For this review, take the finished solid that the model builds, in its own axes (mm). Face numbers are marked on the shaded views. A direction names the side the tool comes from. Round coordinates to 2 decimals unless told otherwise and drop trailing zeros. Order: outer loops, then holes, each group sorted by start corner. A loop starts at its lowest first (then second) coordinate and runs counter-clockwise, first axis right, second up. Notation, with made-up numbers: M -5,-23.5 L 28,-23.5 A16 cw 28,-8.5 Z; hole C 68,84.5 d1. An arc over 180 degrees is marked long. Use a Markdown table: item, result.
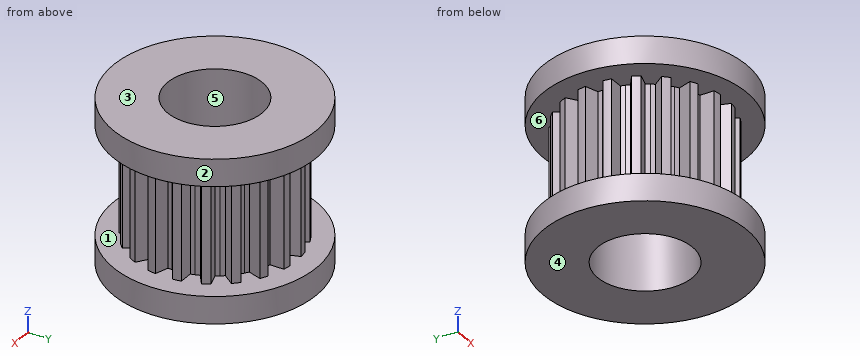
from build123d import *

# Parameters (mm, degrees)
BOSS_EXTRUDE1_DEPTH = 8
SKETCH3_R           = 7.5
BOSS_EXTRUDE2_DEPTH = 2
BOSS_EXTRUDE3_START = 2
SKETCH4_R           = 7.5
BOSS_EXTRUDE3_DEPTH = 2
SKETCH5_R           = 3.5
CUT_EXTRUDE1_DEPTH  = 17.015617378


with BuildPart() as part:
    # Sketch2 → Boss-Extrude1 (new body)
    with BuildSketch(Plane.XY):
        with BuildLine():
            Line((0.323954703, 4.989494298), (0.641126295, 5.965648085))
            ThreePointArc((0.641126295, 5.965648085), (0.93860679, 5.926130044), (1.2337393, 5.871787406))
            Line((1.2337393, 5.871787406), (1.2337393, 4.845398574))
            ThreePointArc((1.2337393, 4.845398574), (1.390142549, 4.802864114), (1.545084972, 4.755282581))
            ThreePointArc((1.545084972, 4.755282581), (1.698403748, 4.702703978), (1.849937763, 4.645183556))
            Line((1.849937763, 4.645183556), (2.453233982, 5.475549564))
            ThreePointArc((2.453233982, 5.475549564), (2.723942998, 5.346039145), (2.987837896, 5.203155264))
            Line((2.987837896, 5.203155264), (2.670666304, 4.227001478))
            ThreePointArc((2.670666304, 4.227001478), (2.806270762, 4.13821754), (2.938926261, 4.045084972))
            ThreePointArc((2.938926261, 4.045084972), (3.068493401, 3.947701641), (3.194836025, 3.846169883))
            Line((3.194836025, 3.846169883), (4.025202033, 4.449466102))
            ThreePointArc((4.025202033, 4.449466102), (4.242640687, 4.242640687), (4.449466102, 4.025202033))
            Line((4.449466102, 4.025202033), (3.846169883, 3.194836025))
            ThreePointArc((3.846169883, 3.194836025), (3.947701641, 3.068493401), (4.045084972, 2.938926261))
            ThreePointArc((4.045084972, 2.938926261), (4.13821754, 2.806270762), (4.227001478, 2.670666304))
            Line((4.227001478, 2.670666304), (5.203155264, 2.987837896))
            ThreePointArc((5.203155264, 2.987837896), (5.346039145, 2.723942998), (5.475549564, 2.453233982))
            Line((5.475549564, 2.453233982), (4.645183556, 1.849937763))
            ThreePointArc((4.645183556, 1.849937763), (4.702703978, 1.698403748), (4.755282581, 1.545084972))
            ThreePointArc((4.755282581, 1.545084972), (4.802864114, 1.390142549), (4.845398574, 1.2337393))
            Line((4.845398574, 1.2337393), (5.871787406, 1.2337393))
            ThreePointArc((5.871787406, 1.2337393), (5.926130044, 0.93860679), (5.965648085, 0.641126295))
            Line((5.965648085, 0.641126295), (4.989494298, 0.323954703))
            ThreePointArc((4.989494298, 0.323954703), (4.997372884, 0.162062503), (5, 0))
            ThreePointArc((5, 0), (4.997372884, -0.162062503), (4.989494298, -0.323954703))
            Line((4.989494298, -0.323954703), (5.965648085, -0.641126295))
            ThreePointArc((5.965648085, -0.641126295), (5.926130044, -0.93860679), (5.871787406, -1.2337393))
            Line((5.871787406, -1.2337393), (4.845398574, -1.2337393))
            ThreePointArc((4.845398574, -1.2337393), (4.802864114, -1.390142549), (4.755282581, -1.545084972))
            ThreePointArc((4.755282581, -1.545084972), (4.702703978, -1.698403748), (4.645183556, -1.849937763))
            Line((4.645183556, -1.849937763), (5.475549564, -2.453233982))
            ThreePointArc((5.475549564, -2.453233982), (5.346039145, -2.723942998), (5.203155264, -2.987837896))
            Line((5.203155264, -2.987837896), (4.227001478, -2.670666304))
            ThreePointArc((4.227001478, -2.670666304), (4.13821754, -2.806270762), (4.045084972, -2.938926261))
            ThreePointArc((4.045084972, -2.938926261), (3.947701641, -3.068493401), (3.846169883, -3.194836025))
            Line((3.846169883, -3.194836025), (4.449466102, -4.025202033))
            ThreePointArc((4.449466102, -4.025202033), (4.242640687, -4.242640687), (4.025202033, -4.449466102))
            Line((4.025202033, -4.449466102), (3.194836025, -3.846169883))
            ThreePointArc((3.194836025, -3.846169883), (3.068493401, -3.947701641), (2.938926261, -4.045084972))
            ThreePointArc((2.938926261, -4.045084972), (2.806270762, -4.13821754), (2.670666304, -4.227001478))
            Line((2.670666304, -4.227001478), (2.987837896, -5.203155264))
            ThreePointArc((2.987837896, -5.203155264), (2.723942998, -5.346039145), (2.453233982, -5.475549564))
            Line((2.453233982, -5.475549564), (1.849937763, -4.645183556))
            ThreePointArc((1.849937763, -4.645183556), (1.698403748, -4.702703978), (1.545084972, -4.755282581))
            ThreePointArc((1.545084972, -4.755282581), (1.390142549, -4.802864114), (1.2337393, -4.845398574))
            Line((1.2337393, -4.845398574), (1.2337393, -5.871787406))
            ThreePointArc((1.2337393, -5.871787406), (0.93860679, -5.926130044), (0.641126295, -5.965648085))
            Line((0.641126295, -5.965648085), (0.323954703, -4.989494298))
            ThreePointArc((0.323954703, -4.989494298), (0.162062503, -4.997372884), (0, -5))
            ThreePointArc((0, -5), (-0.162062503, -4.997372884), (-0.323954703, -4.989494298))
            Line((-0.323954703, -4.989494298), (-0.641126295, -5.965648085))
            ThreePointArc((-0.641126295, -5.965648085), (-0.93860679, -5.926130044), (-1.2337393, -5.871787406))
            Line((-1.2337393, -5.871787406), (-1.2337393, -4.845398574))
            ThreePointArc((-1.2337393, -4.845398574), (-1.390142549, -4.802864114), (-1.545084972, -4.755282581))
            ThreePointArc((-1.545084972, -4.755282581), (-1.698403748, -4.702703978), (-1.849937763, -4.645183556))
            Line((-1.849937763, -4.645183556), (-2.453233982, -5.475549564))
            ThreePointArc((-2.453233982, -5.475549564), (-2.723942998, -5.346039145), (-2.987837896, -5.203155264))
            Line((-2.987837896, -5.203155264), (-2.670666304, -4.227001478))
            ThreePointArc((-2.670666304, -4.227001478), (-2.806270762, -4.13821754), (-2.938926261, -4.045084972))
            ThreePointArc((-2.938926261, -4.045084972), (-3.068493401, -3.947701641), (-3.194836025, -3.846169883))
            Line((-3.194836025, -3.846169883), (-4.025202033, -4.449466102))
            ThreePointArc((-4.025202033, -4.449466102), (-4.242640687, -4.242640687), (-4.449466102, -4.025202033))
            Line((-4.449466102, -4.025202033), (-3.846169883, -3.194836025))
            ThreePointArc((-3.846169883, -3.194836025), (-3.947701641, -3.068493401), (-4.045084972, -2.938926261))
            ThreePointArc((-4.045084972, -2.938926261), (-4.13821754, -2.806270762), (-4.227001478, -2.670666304))
            Line((-4.227001478, -2.670666304), (-5.203155264, -2.987837896))
            ThreePointArc((-5.203155264, -2.987837896), (-5.346039145, -2.723942998), (-5.475549564, -2.453233982))
            Line((-5.475549564, -2.453233982), (-4.645183556, -1.849937763))
            ThreePointArc((-4.645183556, -1.849937763), (-4.702703978, -1.698403748), (-4.755282581, -1.545084972))
            ThreePointArc((-4.755282581, -1.545084972), (-4.802864114, -1.390142549), (-4.845398574, -1.2337393))
            Line((-4.845398574, -1.2337393), (-5.871787406, -1.2337393))
            ThreePointArc((-5.871787406, -1.2337393), (-5.926130044, -0.93860679), (-5.965648085, -0.641126295))
            Line((-5.965648085, -0.641126295), (-4.989494298, -0.323954703))
            ThreePointArc((-4.989494298, -0.323954703), (-4.997372884, -0.162062503), (-5, 0))
            ThreePointArc((-5, 0), (-4.997372884, 0.162062503), (-4.989494298, 0.323954703))
            Line((-4.989494298, 0.323954703), (-5.965648085, 0.641126295))
            ThreePointArc((-5.965648085, 0.641126295), (-5.926130044, 0.93860679), (-5.871787406, 1.2337393))
            Line((-5.871787406, 1.2337393), (-4.845398574, 1.2337393))
            ThreePointArc((-4.845398574, 1.2337393), (-4.802864114, 1.390142549), (-4.755282581, 1.545084972))
            ThreePointArc((-4.755282581, 1.545084972), (-4.702703978, 1.698403748), (-4.645183556, 1.849937763))
            Line((-4.645183556, 1.849937763), (-5.475549564, 2.453233982))
            ThreePointArc((-5.475549564, 2.453233982), (-5.346039145, 2.723942998), (-5.203155264, 2.987837896))
            Line((-5.203155264, 2.987837896), (-4.227001478, 2.670666304))
            ThreePointArc((-4.227001478, 2.670666304), (-4.13821754, 2.806270762), (-4.045084972, 2.938926261))
            ThreePointArc((-4.045084972, 2.938926261), (-3.947701641, 3.068493401), (-3.846169883, 3.194836025))
            Line((-3.846169883, 3.194836025), (-4.449466102, 4.025202033))
            ThreePointArc((-4.449466102, 4.025202033), (-4.242640687, 4.242640687), (-4.025202033, 4.449466102))
            Line((-4.025202033, 4.449466102), (-3.194836025, 3.846169883))
            ThreePointArc((-3.194836025, 3.846169883), (-3.068493401, 3.947701641), (-2.938926261, 4.045084972))
            ThreePointArc((-2.938926261, 4.045084972), (-2.806270762, 4.13821754), (-2.670666304, 4.227001478))
            Line((-2.670666304, 4.227001478), (-2.987837896, 5.203155264))
            ThreePointArc((-2.987837896, 5.203155264), (-2.723942998, 5.346039145), (-2.453233982, 5.475549564))
            Line((-2.453233982, 5.475549564), (-1.849937763, 4.645183556))
            ThreePointArc((-1.849937763, 4.645183556), (-1.698403748, 4.702703978), (-1.545084972, 4.755282581))
            ThreePointArc((-1.545084972, 4.755282581), (-1.390142549, 4.802864114), (-1.2337393, 4.845398574))
            Line((-1.2337393, 4.845398574), (-1.2337393, 5.871787406))
            ThreePointArc((-1.2337393, 5.871787406), (-0.93860679, 5.926130044), (-0.641126295, 5.965648085))
            Line((-0.641126295, 5.965648085), (-0.323954703, 4.989494298))
            ThreePointArc((-0.323954703, 4.989494298), (-0.162062503, 4.997372884), (0, 5))
            ThreePointArc((0, 5), (0.162062503, 4.997372884), (0.323954703, 4.989494298))
        make_face()
    extrude(amount=BOSS_EXTRUDE1_DEPTH)

    # Sketch3 → Boss-Extrude2 (add)
    with BuildSketch(Plane.XY.offset(8)):
        Circle(SKETCH3_R)
    extrude(amount=BOSS_EXTRUDE2_DEPTH)

    # Sketch4 → Boss-Extrude3 (add)
    with BuildSketch(Plane(origin=(0, 0, 0), x_dir=(-1, 0, 0), z_dir=(0, 0, -1)).offset(BOSS_EXTRUDE3_START)):
        with Locations(Location((0, 0, 0), (0, 0, 180))):
            Circle(SKETCH4_R)
    extrude(amount=-BOSS_EXTRUDE3_DEPTH)

    # Sketch5 → Cut-Extrude1 (cut, through all)
    with BuildSketch(Plane(origin=(0, 0, -2), x_dir=(-1, 0, 0), z_dir=(0, 0, -1))):
        Circle(SKETCH5_R)
    extrude(amount=-CUT_EXTRUDE1_DEPTH, mode=Mode.SUBTRACT)


solid = part.part
Q1. Add section A-A (z = 8.25). Write out the cut boundary in (x, y).
Determined:
| item | result |
|---|---|
| outline | C 0,0 d15; hole C 0,0 d7 |
Q2. Wall thickness on line 1 along Z through (x, y) = (-1.75, 7); line 2 along Y through (x, z) = (-4, 0.5); line 3 along Y through (x, z) = (0, 8.25): over which ranges is each line inside the solid? List them lowest first. Write a range as [from, to].
Determined:
| item | result |
|---|---|
| line 1 | z = [-2, 0], [8, 10] |
| line 2 | y = [-4.43, -3.41], [-3, 3], [3.41, 4.43] |
| line 3 | y = [-7.5, -3.5], [3.5, 7.5] |
Q3. Machinability: for the marked faces 5 and 6, which of the approach directions +Z, -Z, +X, -X, +Y, -Y give a long, thin tool a straight path to every point of the face, cutting with its end or side? Answer none if there is none.
Determined:
| item | result |
|---|---|
| face 5 | +Z, -Z |
| face 6 | none |
Q4. Add section B-B (y = 6.75). Write out the cut boundary in (x, z).
Determined:
| item | result |
|---|---|
| outline | M -3.27,-2 L 3.27,-2 L 3.27,0 L -3.27,0 Z; M -3.27,8 L 3.27,8 L 3.27,10 L -3.27,10 Z |
Q5. Draft analysis for pull direction Z (two halves, no side actions). For the marked faces 1, 2, 3 and 4, state which applies: pulls with the +Z half, pulls with the -Z half, needs draft (parallel to the pull), parting line crosses it, or undercut.
Determined:
| item | result |
|---|---|
| face 1 | undercut |
| face 2 | needs draft |
| face 3 | pulls with the +Z half |
| face 4 | pulls with the -Z half |
Q6. Clearance check with flat-ended pins moving along their axes: pin 1 (1.1 mm diameter, centred on x = -5.5, z = 5.5, fed in from -Y); pin 2 (0.8 mm diameter, centred on y = 5, z = 4.5, fed in from +X); pin 3 (1.5 mm diameter, centred on x = 4.5, z = -0.5, fed in from +Y). State where each tip first meets the part, or that it passes through.
Determined:
| item | result |
|---|---|
| pin 1 | stops at y = -2.99 |
| pin 2 | stops at x = 2.99 |
| pin 3 | stops at y = 6.5 |
